Source: CAD feature listing. Evaluate the final solid. Frame: model axes, mm. A direction names the side the tool comes from. Round coordinates to 2 decimals unless told otherwise and drop trailing zeros. Order: outer loops, then holes, each group sorted by start corner. A loop starts at its lowest first (then second) coordinate and runs counter-clockwise, first axis right, second up. Notation, with made-up numbers: M 6,36.25 L 19,36.25 A22 ccw 19,59.25 Z; hole C 40.25,71 d2. An arc over 180 degrees is marked long. Use one line per item in the form item = value. Start each with the question number.
Q1. Contact query for flat-ended pins moving along their axis: pin 1 (3 mm diameter, centred on y = -1, z = -3, fed in from -X); pin 2 (1.9 mm diameter, centred on y = 0, z = 5, fed in from +X). Output: stop coordinate, or through.
Q2. Material intervals for probe 1 along Y at (x, z) = (7.5, -4); probe 2 along Z at (x, y) = (6.5, -2); probe 3 along Z at (x, y) = (3.5, -1.25), sorted ascending.
Q3. Section A-A (z = 5). Return the cut outline in (x, y), plus the area to 3 significant figures.
Q4. Section B-B (x = 5.5). Return the cut outline in (y, z), plus the area to 3 significant figures.
Q5. Section D-D (y = -1.5). Give the number of separate pieces and of enclosed holes in the cut face, plus the area to 3 significant figures.
Q6. Reachability of faces 1 (the cylindrical face through (7.406, 0.946, -7.005)), 2 (the cylindrical face through (3.958, 0.751, -6.385)), 3 (the flat face through (1, 2, -2)) from +Z, -Z, +X, -X, +Y, -Y: full face, straight path, thin tool, end or side. Return the list, or none.
Q7. Section C-C (z = -3.5). Return the cut outline in (x, y).
Q8. Pull-direction query (Z, two-part tool) for faces 4 (the cylindrical face through (1, 0, -0.3)), 5 (the cylindrical face through (3.8, 0.1, -7.7)), 6 (the cylindrical face through (3.8, -0.1, 7.7)), 7 (the flat face through (4, 3.7, 0)); classes: pulls with the +Z half, pulls with the -Z half, needs draft (parallel to the pull), parting line crosses it, or undercut.
from build123d import *

# Parameters (mm, degrees)
EXTRUDE_1_DEPTH          = 7.8
CUT_EXTRUDE_1_DEPTH      = 12.568059474
CUT_EXTRUDE_1_DEPTH_BACK = 12.568059474
SKETCH_2_3_R             = 2.5
SKETCH_2_6_R             = 3.15
CUT_EXTRUDE_6_DEPTH      = 1
CUT_EXTRUDE_START        = -2
CUT_EXTRUDE_7_DEPTH      = 2
CUT_EXTRUDE_START_2      = -7.8
CUT_EXTRUDE_8_DEPTH      = 2


with BuildPart() as part:
    # 草图2 → 凸台-拉伸1 (new body)
    with BuildSketch(Plane(origin=(0, 0, 0), x_dir=(0, 0, -1), z_dir=(1, 0, 0))):
        with BuildLine():
            Line((-4, 3.7), (4, 3.7))
            ThreePointArc((4, 3.7), (7.7, 0), (4, -3.7))
            Line((4, -3.7), (-4, -3.7))
            ThreePointArc((-4, -3.7), (-7.7, 0), (-4, 3.7))
        make_face()
    extrude(amount=EXTRUDE_1_DEPTH)

    # 草图2<3> → 切除-拉伸1 (cut, two sides: drawn at the far end of the back side and taken through both)
    with BuildSketch(Plane(origin=(0, 0, 0), x_dir=(0, 0, -1), z_dir=(1, 0, 0)).offset(-CUT_EXTRUDE_1_DEPTH_BACK)):
        with Locations((-4, 0)):
            Circle(SKETCH_2_3_R)
        with Locations((4, 0)):
            Circle(SKETCH_2_3_R)
    extrude(amount=CUT_EXTRUDE_1_DEPTH + CUT_EXTRUDE_1_DEPTH_BACK, mode=Mode.SUBTRACT)

    # 草图2<6> → 切除-拉伸6 (cut)
    with BuildSketch(Plane(origin=(0, 0, 0), x_dir=(0, 0, -1), z_dir=(1, 0, 0))):
        with Locations((-4, 0)):
            Circle(SKETCH_2_6_R)
        with Locations((4, 0)):
            Circle(SKETCH_2_6_R)
    cut_extrude_6 = extrude(amount=CUT_EXTRUDE_6_DEPTH, mode=Mode.SUBTRACT)

    # 镜向1: 切除-拉伸6 across plane
    add(cut_extrude_6.mirror(Plane(origin=(4, 0, 0), x_dir=(0, 0, 1), z_dir=(1, 0, 0))), mode=Mode.SUBTRACT)

    # 草图3 → 切除-拉伸7 (cut)
    with BuildSketch(Plane(origin=(7.8, 0, 0), x_dir=(0, 0, -1), z_dir=(1, 0, 0)).offset(CUT_EXTRUDE_START)):
        with BuildLine():
            Line((1.610570152, 2.825), (-1.610570152, 2.825))
            ThreePointArc((-1.610570152, 2.825), (-0.643596386, 1.557098192), (-0.3, 0))
            ThreePointArc((-0.3, 0), (-0.643596386, -1.557098192), (-1.610570152, -2.825))
            Line((-1.610570152, -2.825), (1.610570152, -2.825))
            ThreePointArc((1.610570152, -2.825), (0.3, 0), (1.610570152, 2.825))
        make_face()
    extrude(amount=CUT_EXTRUDE_7_DEPTH, mode=Mode.SUBTRACT)

    # 草图3<3> → 切除-拉伸8 (cut)
    with BuildSketch(Plane(origin=(7.8, 0, 0), x_dir=(0, 0, -1), z_dir=(1, 0, 0)).offset(CUT_EXTRUDE_START_2)):
        with BuildLine():
            Line((1.610570152, 2.825), (-1.610570152, 2.825))
            ThreePointArc((-1.610570152, 2.825), (-0.643596386, 1.557098192), (-0.3, 0))
            ThreePointArc((-0.3, 0), (-0.643596386, -1.557098192), (-1.610570152, -2.825))
            Line((-1.610570152, -2.825), (1.610570152, -2.825))
            ThreePointArc((1.610570152, -2.825), (0.3, 0), (1.610570152, 2.825))
        make_face()
    extrude(amount=CUT_EXTRUDE_8_DEPTH, mode=Mode.SUBTRACT)


solid = part.part
Results list:
q1.pin_1 = 1
q1.pin_2 = through
q2.probe_1 = -3.7 to -3.15, 3.15 to 3.7
q2.probe_2 = -7.11 to -5.5, -2.5 to -0.89, 0.89 to 2.5, 5.5 to 7.11
q2.probe_3 = -7.48 to -6.17, -1.83 to 1.83, 6.17 to 7.48
q3.outline = M 0,-3.56 L 7.8,-3.56 L 7.8,-2.99 L 7,-2.99 L 7,-2.29 L 1,-2.29 L 1,-2.99 L 0,-2.99 Z; M 0,2.99 L 1,2.99 L 1,2.29 L 7,2.29 L 7,2.99 L 7.8,2.99 L 7.8,3.56 L 0,3.56 Z
q3.area = 17.3 mm2
q4.outline = M -3.7,-4 A3.7 ccw 3.7,-4 L 3.7,4 A3.7 ccw -3.7,4 Z; hole C 0,-4 d5; hole C 0,4 d5
q4.area = 62.9 mm2
q5.separate_pieces = 3
q5.enclosed_holes = 0
q5.area = 42.3 mm2
q6.face_1 = +X
q6.face_2 = +X, -X
q6.face_3 = -X
q7.outline = M 0,-3.7 L 7.8,-3.7 L 7.8,-3.11 L 7,-3.11 L 7,-2.45 L 1,-2.45 L 1,-3.11 L 0,-3.11 Z; M 0,3.11 L 1,3.11 L 1,2.45 L 7,2.45 L 7,3.11 L 7.8,3.11 L 7.8,3.7 L 0,3.7 Z
q8.face_4 = undercut
q8.face_5 = pulls with the -Z half
q8.face_6 = pulls with the +Z half
q8.face_7 = needs draft
